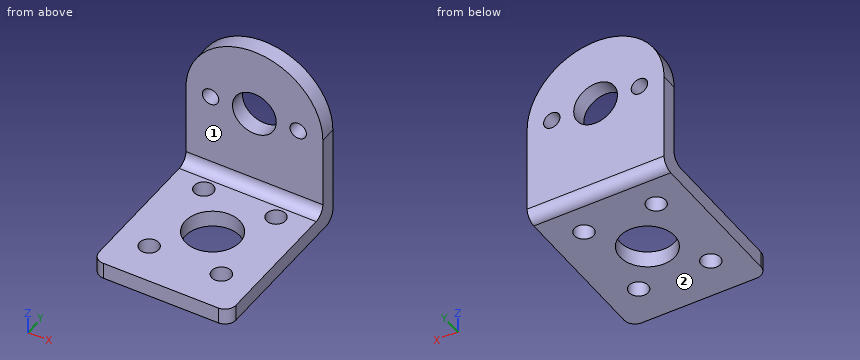
from build123d import *

# Parameters (mm, degrees)
ESQUISSE1_W             = 25
ESQUISSE1_H             = 31
ESQUISSE1_R             = 5
ESQUISSE1_R_2           = 1.75
BOSS_EXTRU_1_DEPTH      = 3
ESQUISSE2_W             = 25
ESQUISSE2_H             = 3
BOSS_EXTRU_2_DEPTH      = 30
ESQUISSE3_R             = 4
ESQUISSE3_R_2           = 1.5
ENL_V_MAT_EXTRU_1_DEPTH = 30
CONG_1_R                = 2


with BuildPart() as part:
    # Esquisse1 → Boss.-Extru.1 (new body)
    with BuildSketch(Plane.XY):
        with Locations((12.5, -0.075620767)):
            Rectangle(ESQUISSE1_W, ESQUISSE1_H)
        with Locations((12.5, -0.075620767)):
            Circle(ESQUISSE1_R, mode=Mode.SUBTRACT)
        with Locations((19.091400737, 8.097716147)):
            Circle(ESQUISSE1_R_2, mode=Mode.SUBTRACT)
        with Locations(Location((5.908599263, 8.097716147, 0), (0, 0, 180))):
            Circle(ESQUISSE1_R_2, mode=Mode.SUBTRACT)
        with Locations(Location((19.091400737, -8.248957682, 0), (0, 0, 180))):
            Circle(ESQUISSE1_R_2, mode=Mode.SUBTRACT)
        with Locations((5.908599263, -8.248957682)):
            Circle(ESQUISSE1_R_2, mode=Mode.SUBTRACT)
    extrude(amount=BOSS_EXTRU_1_DEPTH)

    # Esquisse2 → Boss.-Extru.2 (add)
    with BuildSketch(Plane.XY.offset(3)):
        with Locations((12.5, 13.924379233)):
            Rectangle(ESQUISSE2_W, ESQUISSE2_H)
    extrude(amount=BOSS_EXTRU_2_DEPTH)

    # Esquisse3 → Enlèv. mat.-Extru.1 (cut)
    with BuildSketch(Plane.XZ.offset(-12.424379233)):
        with Locations((12.5, 18)):
            Circle(ESQUISSE3_R)
        with Locations((20.5, 18)):
            Circle(ESQUISSE3_R_2)
        with Locations(Location((4.5, 18, 0), (0, 0, 270))):
            Circle(ESQUISSE3_R_2)
        with BuildLine():
            Line((0, 18.000546853), (0, 33))
            Line((0, 33), (25.000000024, 33))
            Line((25.000000024, 33), (25.000000024, 18.000546853))
            ThreePointArc((25.000000024, 18.000546853), (12.500000012, 30.500546865), (0, 18.000546853))
        make_face()
    extrude(amount=-ENL_V_MAT_EXTRU_1_DEPTH, mode=Mode.SUBTRACT)

    # Congé1
    cong_1_edges = [part.edges().sort_by_distance(p)[0] for p in [
        (12.5, 12.424379233, 3),
        (12.5, 15.424379233, 0),
        (25, -15.575620767, 1.5),
        (0, -15.575620767, 1.5),
    ]]
    fillet(cong_1_edges, radius=CONG_1_R)


solid = part.part
Input: part model. Units: mm. Frame: model coordinates. Face numbers are marked on the shaded views. A direction names the side the tool comes from. Round coordinates to 2 decimals unless told otherwise and drop trailing zeros. Order: outer loops, then holes, each group sorted by start corner. A loop starts at its lowest first (then second) coordinate and runs counter-clockwise, first axis right, second up.
1. Material intervals for line 1 (Z direction, x = 12.5, y = 13.55); line 2 (Y direction, x = 9, z = 16); line 3 (Z direction, x = 21.25, y = -1.5), sorted ascending.
The answers:
line 1: z = 0 to 14, 22 to 30.5
line 2: y = 12.42 to 15.42
line 3: z = 0 to 3
2. Pin query (flat end, axial travel): P1, Ø3, axis at x = 5.91, y = -8.25, coming from the -Z side; P2, Ø7.5, axis at x = 11, y = -7, coming from the +Z side; P3, Ø12.5, axis at x = 13, z = 16, coming from the -Y side; P4, Ø6, axis at x = 6.5, y = 10.5, coming from the +Z side. Return the tip coordinate at first contact, or that it passes through.
The answers:
P1: passes through
P2: stops at z = 3
P3: stops at y = 12.42
P4: stops at z = 29.94
3. Cut plane D-D, the plane z = 14.5. Output: boundary loops of the cut face in (x, y), then the cut area to 3 significant figures.
The answers:
outline: (0, 12.42) - (10.56, 12.42) - (10.56, 15.42) - (0, 15.42) - close; (14.44, 12.42) - (25, 12.42) - (25, 15.42) - (14.44, 15.42) - close
area: 63.4 mm2
4. Cut plane C-C, the plane y = 13. Output: boundary loops of the cut face in (x, z), then the cut area to 3 significant figures.
The answers:
outline: (0, 0) - (25, 0) - (25, 18) arc R12.5 ccw to (0, 18) - close; hole circle Ø3 at (4.5, 18); hole circle Ø8 at (12.5, 18); hole circle Ø3 at (20.5, 18)
area: 631 mm2
5. Cut plane B-B, the plane y = 0.5. Output: boundary loops of the cut face in (x, z).
The answers:
outline: (0, 0) - (7.53, 0) - (7.53, 3) - (0, 3) - close; (17.47, 0) - (25, 0) - (25, 3) - (17.47, 3) - close
6. Cut plane A-A, the plane x = 12.5. Output: boundary loops of the cut face in (y, z).
The answers:
outline: (-15.58, 0) - (-5.08, 0) - (-5.08, 3) - (-15.58, 3) - close; (4.92, 0) - (13.42, 0) arc R2 ccw to (15.42, 2) - (15.42, 14) - (12.42, 14) - (12.42, 5) arc R2 cw to (10.42, 3) - (4.92, 3) - close; (12.42, 22) - (15.42, 22) - (15.42, 30.5) - (12.42, 30.5) - close
7. Set-up query: the marked faces 1 and 2. Return all of +Z, -Z, +X, -X, +Y, -Y with unobstructed straight access to the full face (end or side cutting, diameter ignored); none if empty.
The answers:
face 1: +Z, +X, -X, -Y
face 2: -Z, +X, -X, +Y, -Y
